Autodesk Fusion 360 part; units mm, degrees
sketch "Sketch1" plane through (0, 0, 0) normal (0, 0, 1) x (1, 0, 0)
  circle A0 centre (0, 5) radius 1.75
  line L0 (-7, 6.5) -> (7, 6.5)
  line L1 (7, 6.5) -> (7, 0)
  line L2 (7, 0) -> (-7, 0)
  line L3 (-7, 0) -> (-7, 6.5)
  line L4 (0, 2.5) -> (0, 20) construction
  dimension "d1" = 3.5
  dimension "d2" = 5
  dimension "d3" = 14
  dimension "d4" = 6.5
extrude "Extrude1" add sketch "Sketch1" against normal blind 4 contours A0 L0 L1 L2 L3
sketch "Sketch3" plane through (0, 6.5, 0) normal (0, 1, 0) x (-1, 0, 0)
  line L0 (-0.9014, 0) -> (-7, 0)
  line L1 (-7, 0) -> (-7, -4)
  line L2 (-7, -4) -> (-0.9014, -4)
  line L3 (7, -4) -> (7, 0)
  line L4 (7, -2) -> (-7, -2) construction
  line L5 (0, 0) -> (0, -4.5) construction
  line L6 (-0.9014, -4) -> (-0.9014, 0)
  line L7 (7, 0) -> (0.9014, 0)
  line L8 (0.9014, 0) -> (0.9014, -4)
  line L9 (0.9014, -4) -> (7, -4)
  point P0 (5, -2)
  point P1 (-5, -2)
  dimension "d7" = 10
hole "Hole1" at (5, 6.5, -2) at (-5, 6.5, -2) direction (0, -1, 0) diameter 2.2 end through all countersink diameter 4.4 countersink angle 90
hole "Hole2" at (0, 0, -2) direction (0, 1, 0) diameter 1.875 depth 7.5 tip angle 118
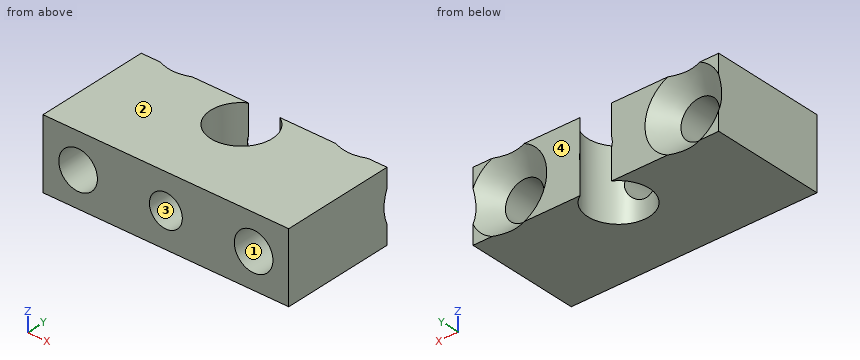
Model file for the job. Use its own axes, mm. Face numbers are marked on the shaded views. Give positions to 0.01 mm unless a question says otherwise; leave off trailing zeros. Order: outer loops, then holes, each group sorted by start corner. A loop starts at its lowest first (then second) coordinate and runs counter-clockwise, first axis right, second up.
1) Saw through at B-B, the plane x = 0. Write the cut outline in (y, z), then the cut area to 3 significant figures.
2) Saw through at A-A, the plane y = 5. Write the cut outline in (x, z), then the cut area to 3 significant figures.
3) Saw through at D-D, the plane x = 5. Write the cut outline in (y, z).
4) Saw through at C-C, the plane y = 2.25. Write the cut outline in (x, z) (1 decimal).
5) Pin check, flat tips, straight feed: pin 1 (2 mm diameter, centred on x = 5, z = -2, fed in from +Y); pin 2 (1 mm diameter, centred on x = -4, z = -3, fed in from +Y). Stop position of each tip, or through.
6) Wall check: probe 1 along X at (y, z) = (2.6, -2); probe 2 along Z at (x, y) = (-5, 2.6); probe 3 along Z at (x, y) = (0, 1.55). Give the ranges that are in metal, low to high.
7) Mould opens along Z. For the marked faces 1, 2, 3 and 4 say: +Z half, -Z half, draft (parallel to the pull), parting line (faces both ways), or undercut.
Computed:
1. outline: (0, -4) - (3.25, -4) - (3.25, -2.94) - (0, -2.94) - close; (0, -1.06) - (3.25, -1.06) - (3.25, 0) - (0, 0) - close
1. area: 6.91 mm2
2. outline: (-7, -4) - (-1.75, -4) - (-1.75, 0) - (-7, 0) - close; (1.75, -4) - (7, -4) - (7, 0) - (1.75, 0) - close; hole circle Ø2.2 at (-5, -2); hole circle Ø2.2 at (5, -2)
2. area: 34.4 mm2
3. outline: (0, -4) - (6.3, -4) - (5.4, -3.1) - (0, -3.1) - close; (0, -0.9) - (5.4, -0.9) - (6.3, 0) - (0, 0) - close
4. outline: (-7, -4) - (7, -4) - (7, 0) - (-7, 0) - close; hole circle Ø2.2 at (-5, -2); hole circle Ø1.9 at (0, -2); hole circle Ø2.2 at (5, -2)
5. pin 1: passes through
5. pin 2: stops at y = 6.21
6. probe 1: x = -7 to -6.1, -3.9 to -0.94, 0.94 to 3.9, 6.1 to 7
6. probe 2: z = -4 to -3.1, -0.9 to 0
6. probe 3: z = -4 to -2.94, -1.06 to 0
7. face 1: undercut
7. face 2: +Z half
7. face 3: undercut
7. face 4: draft
